The listing builds one solid part. Answer for the finished solid, in the listing's coordinates (mm). A direction names the side the tool comes from. Coordinates: 2 decimals unless noted, no trailing zeros. Loops run counter-clockwise (first coordinate to the right, second up) from the corner with the lowest first, then second, coordinate; pieces in that order, holes last. Notation, with made-up numbers: M 17,18 L 37,18 A14 ccw 37,25 Z; hole C -2,42 d1. An arc over 180 degrees is marked long. Answer as a JSON object with one key per item and string values. Group by question number.
1. A cutting plane is placed at B-B on y = 29.5. State how many separate pieces and enclosed holes the cut face has, and give its area (3 significant figures).
2. A cutting plane is placed at A-A on z = 18.5. Give the vertices of the cut face in (x, y), and give its area (3 significant figures).
3. Straight lines are drawn through the part: L1, parallel to X at y = 26.5, z = 9; L2, parallel to X at y = -19.5, z = 7.75 (1 decimal); L3, parallel to Y at x = -25, z = 1.75. For each, find the intervals that lie inside material, in ascending order.
4. For faces 1 (the face through (-14, 25, 2)), 2 (the face through (23.5, 0, 1)), determine the directions among +Z, -Z, +X, -X, +Y, -Y from which every point of the face is accessible in a straight line to the end or side of a thin tool.
5. Given pin 1 (1.5 mm diameter, centred on x = 16.5, z = 3.5, fed in from -Y); pin 2 (2.5 mm diameter, centred on x = 14, y = 23, fed in from -Z); pin 3 (5 mm diameter, centred on x = 21.5, y = -19.5, fed in from +Z); pin 4 (3 mm diameter, centred on x = 20.5, y = 2.5, fed in from -Z), each flat-ended and moving along its own axis, determine where each tip first touches the part or whether it passes through.
from build123d import *

# Parameters (mm, degrees)
SKETCH1_R                = 31.75
BOSS_EXTRUDE1_DEPTH      = 13
FILLET1_R                = 5
SHELL1_T                 = -1.5
SKETCH9_R                = 35.624492326
SKETCH9_R_2              = 27.25
BOSS_EXTRUDE5_DEPTH      = 2
SKETCH2_W                = 7.351458637
SKETCH2_H                = 15
BOSS_EXTRUDE2_DEPTH      = 2
BOSS_EXTRUDE3_REACH      = 59.839
SKETCH4_W                = 10.926622009
SKETCH4_H                = 2.5
FILLET3_R                = 1
BOSS_EXTRUDE4_REACH      = 60.696
BOSS_EXTRUDE4_END_RADIUS = 38.178049598
SKETCH5_W                = 10.787818312
SKETCH5_H                = 8
SKETCH6_W                = 2
SKETCH6_H                = 4
CUT_EXTRUDE1_DEPTH       = 4
SKETCH7_W                = 4
SKETCH7_H                = 2
CUT_EXTRUDE2_DEPTH       = 4
SKETCH8_W                = 4
SKETCH8_H                = 2
CUT_EXTRUDE3_DEPTH       = 4
FILLET5_R                = 1
CHAMFER2_SIZE            = 1.5
FILLET7_R                = 1
CHAMFER3_SIZE            = 0.5


with BuildPart() as part:
    # Sketch1 → Boss-Extrude1 (new body)
    with BuildSketch(Plane.XY):
        with Locations(Location((0, 0, 0), (0, 0, 180))):
            Circle(SKETCH1_R)
    extrude(amount=BOSS_EXTRUDE1_DEPTH)

    # Fillet1
    fillet1_edges = [part.edges().sort_by_distance(p)[0] for p in [
        (31.75, 0, 13),
    ]]
    fillet(fillet1_edges, radius=FILLET1_R)

    # Sketch12 → Revolve3 (revolve)
    with BuildSketch(Plane(origin=(0, 0, 0), x_dir=(1, 0, 0), z_dir=(0, 1, 0)), mode=Mode.PRIVATE) as revolve3_sk:
        with BuildLine():
            Line((0, -25.950011953), (0, -11.6))
            Line((0, -11.6), (27.242806288, -11.6))
            Line((27.242806288, -11.6), (27.242806288, -11.107193712))
            ThreePointArc((27.242806288, -11.107193712), (29.439924032, -10.197117744), (30.35, -8))
            Line((30.35, -8), (30.35, 0))
            Line((30.35, 0), (37.227524794, 0))
            ThreePointArc((37.227524794, 0), (22.689709797, -18.822303202), (0, -25.950011953))
        make_face()
    revolve(revolve3_sk.sketch.rotate(Axis((0, 0, 27.247512551), (0, 0, -1)), 180), axis=Axis((0, 0, 27.247512551), (0, 0, -1)))

    # Shell1
    shell1_openings = [part.faces().sort_by_distance(p)[0] for p in [
        (0, 0, 0),
    ]]
    offset(amount=SHELL1_T, openings=shell1_openings, kind=Kind.INTERSECTION)

    # Sketch9 → Boss-Extrude5 (add)
    with BuildSketch(Plane(origin=(0, 0, 0), x_dir=(-1, 0, 0), z_dir=(0, 0, -1))):
        Circle(SKETCH9_R)
        Circle(SKETCH9_R_2, mode=Mode.SUBTRACT)
    extrude(amount=-BOSS_EXTRUDE5_DEPTH)

    # Sketch2 → Boss-Extrude2 (add)
    with BuildSketch(Plane(origin=(0, 0, 0), x_dir=(-1, 0, 0), z_dir=(0, 0, -1))):
        with Locations((-27.175729319, 0)):
            Rectangle(SKETCH2_W, SKETCH2_H)
        Polygon((8.93053879, 30.468146923), (5.254809472, 24.101596989), (18.245190528, 16.601596989), (21.920919847, 22.968146923), align=None)
        Polygon((21.920919847, -22.968146923), (18.245190528, -16.601596989), (5.254809472, -24.101596989), (8.93053879, -30.468146923), align=None)
    extrude(amount=-BOSS_EXTRUDE2_DEPTH)

    # Sketch4 → Boss-Extrude3 (add, up to next)
    with BuildSketch(Plane.XY.offset(2), mode=Mode.PRIVATE) as boss_extrude3_sk1:
        with Locations((28.963311004, 6.25)):
            Rectangle(SKETCH4_W, SKETCH4_H)
    boss_extrude3_tool1 = extrude(boss_extrude3_sk1.sketch, amount=BOSS_EXTRUDE3_REACH, mode=Mode.PRIVATE) - part.part
    # Sketch4 → Boss-Extrude3 (add, up to next)
    with BuildSketch(Plane.XY.offset(2), mode=Mode.PRIVATE) as boss_extrude3_sk2:
        with Locations((28.963311004, -6.25)):
            Rectangle(SKETCH4_W, SKETCH4_H)
    boss_extrude3_tool2 = extrude(boss_extrude3_sk2.sketch, amount=BOSS_EXTRUDE3_REACH, mode=Mode.PRIVATE) - part.part
    # Sketch4 → Boss-Extrude3 (add, up to next)
    with BuildSketch(Plane.XY.offset(2), mode=Mode.PRIVATE) as boss_extrude3_sk3:
        Polygon((-16.080127019, -17.851596989), (-21.543438023, -27.314329226), (-23.708501533, -26.064329226), (-18.245190528, -16.601596989), align=None)
    boss_extrude3_tool3 = extrude(boss_extrude3_sk3.sketch, amount=BOSS_EXTRUDE3_REACH, mode=Mode.PRIVATE) - part.part
    # Sketch4 → Boss-Extrude3 (add, up to next)
    with BuildSketch(Plane.XY.offset(2), mode=Mode.PRIVATE) as boss_extrude3_sk4:
        Polygon((-7.419872981, -22.851596989), (-12.883183985, -32.314329226), (-10.718120476, -33.564329226), (-5.254809472, -24.101596989), align=None)
    boss_extrude3_tool4 = extrude(boss_extrude3_sk4.sketch, amount=BOSS_EXTRUDE3_REACH, mode=Mode.PRIVATE) - part.part
    # Sketch4 → Boss-Extrude3 (add, up to next)
    with BuildSketch(Plane.XY.offset(2), mode=Mode.PRIVATE) as boss_extrude3_sk5:
        Polygon((-7.419872981, 22.851596989), (-12.883183985, 32.314329226), (-10.718120476, 33.564329226), (-5.254809472, 24.101596989), align=None)
    boss_extrude3_tool5 = extrude(boss_extrude3_sk5.sketch, amount=BOSS_EXTRUDE3_REACH, mode=Mode.PRIVATE) - part.part
    # Sketch4 → Boss-Extrude3 (add, up to next)
    with BuildSketch(Plane.XY.offset(2), mode=Mode.PRIVATE) as boss_extrude3_sk6:
        Polygon((-16.080127019, 17.851596989), (-21.543438023, 27.314329226), (-23.708501533, 26.064329226), (-18.245190528, 16.601596989), align=None)
    boss_extrude3_tool6 = extrude(boss_extrude3_sk6.sketch, amount=BOSS_EXTRUDE3_REACH, mode=Mode.PRIVATE) - part.part
    add(boss_extrude3_tool1.solids().sort_by_distance((28.963311, 6.25, 2))[0])
    add(boss_extrude3_tool2.solids().sort_by_distance((28.963311, -6.25, 2))[0])
    add(boss_extrude3_tool3.solids().sort_by_distance((-19.894314, -21.957963, 2))[0])
    add(boss_extrude3_tool4.solids().sort_by_distance((-9.068997, -28.207963, 2))[0])
    add(boss_extrude3_tool5.solids().sort_by_distance((-9.068997, 28.207963, 2))[0])
    add(boss_extrude3_tool6.solids().sort_by_distance((-19.894314, 21.957963, 2))[0])

    # Fillet3
    fillet3_edges = [part.edges().sort_by_distance(p)[0] for p in [
        (23.5, -7.5, 7.705328032),
        (23.5, 7.5, 7.705328032),
        (-5.254809472, 24.101596989, 7.705328032),
        (-18.245190528, 16.601596989, 7.705328032),
        (-18.245190528, -16.601596989, 7.705328032),
        (-5.254809472, -24.101596989, 7.705328032),
    ]]
    fillet(fillet3_edges, radius=FILLET3_R)

    # Boss-Extrude4: up to this sphere (the profile starts inside it)
    boss_extrude4_end = Location((0, 0, -13.728037644)) * Sphere(BOSS_EXTRUDE4_END_RADIUS, mode=Mode.PRIVATE)
    # Sketch5 → Boss-Extrude4 (add, up to the surface)
    with BuildSketch(Plane(origin=(0, 0, 0), x_dir=(-1, 0, 0), z_dir=(0, 0, -1)), mode=Mode.PRIVATE) as boss_extrude4_sk1:
        with Locations((29.393909156, 0)):
            Rectangle(SKETCH5_W, SKETCH5_H)
    boss_extrude4_tool1 = extrude(boss_extrude4_sk1.sketch, amount=-BOSS_EXTRUDE4_REACH, mode=Mode.PRIVATE) & boss_extrude4_end
    add(boss_extrude4_tool1.solids().sort_by_distance((-29.393909, 0, 0))[0])
    # Sketch5 → Boss-Extrude4 (add, up to the surface)
    with BuildSketch(Plane(origin=(0, 0, 0), x_dir=(-1, 0, 0), z_dir=(0, 0, -1)), mode=Mode.PRIVATE) as boss_extrude4_sk2:
        Polygon((-8.535898385, -22.784609691), (-15.464101615, -18.784609691), (-20.858010771, -28.127134401), (-13.929807541, -32.127134401), align=None)
    boss_extrude4_tool2 = extrude(boss_extrude4_sk2.sketch, amount=-BOSS_EXTRUDE4_REACH, mode=Mode.PRIVATE) & boss_extrude4_end
    add(boss_extrude4_tool2.solids().sort_by_distance((14.696955, -25.455872, 0))[0])
    # Sketch5 → Boss-Extrude4 (add, up to the surface)
    with BuildSketch(Plane(origin=(0, 0, 0), x_dir=(-1, 0, 0), z_dir=(0, 0, -1)), mode=Mode.PRIVATE) as boss_extrude4_sk3:
        Polygon((-15.464101615, 18.784609691), (-8.535898385, 22.784609691), (-13.929807541, 32.127134401), (-20.858010771, 28.127134401), align=None)
    boss_extrude4_tool3 = extrude(boss_extrude4_sk3.sketch, amount=-BOSS_EXTRUDE4_REACH, mode=Mode.PRIVATE) & boss_extrude4_end
    add(boss_extrude4_tool3.solids().sort_by_distance((14.696955, 25.455872, 0))[0])

    # Sketch6 → Cut-Extrude1 (cut)
    with BuildSketch(Plane(origin=(-24, 0, 0), x_dir=(0, 0, -1), z_dir=(1, 0, 0))):
        with Locations((-6, 0)):
            Rectangle(SKETCH6_W, SKETCH6_H)
    extrude(amount=-CUT_EXTRUDE1_DEPTH, mode=Mode.SUBTRACT)

    # Sketch7 → Cut-Extrude2 (cut)
    with BuildSketch(Plane(origin=(12, -20.784609691, 0), x_dir=(0.8660254037844365, 0.5000000000000039, 0), z_dir=(-0.5000000000000038, 0.8660254037844364, 0))):
        with Locations((0, -6)):
            Rectangle(SKETCH7_W, SKETCH7_H)
    extrude(amount=-CUT_EXTRUDE2_DEPTH, mode=Mode.SUBTRACT)

    # Sketch8 → Cut-Extrude3 (cut)
    with BuildSketch(Plane(origin=(12, 20.784609691, 0), x_dir=(0.8660254037844257, -0.5000000000000224, 0), z_dir=(-0.5000000000000224, -0.8660254037844258, 0))):
        with Locations((0, 6)):
            Rectangle(SKETCH8_W, SKETCH8_H)
    extrude(amount=-CUT_EXTRUDE3_DEPTH, mode=Mode.SUBTRACT)

    # Fillet5
    fillet5_edges = [part.edges().sort_by_distance(p)[0] for p in [
        (-24, -4, 7.846211216),
        (-24, 4, 7.846211216),
        (15.464101615, -18.784609691, 7.846211216),
        (8.535898385, -22.784609691, 7.846211216),
        (8.535898385, 22.784609691, 7.846211216),
        (15.464101615, 18.784609691, 7.846211216),
    ]]
    fillet(fillet5_edges, radius=FILLET5_R)

    # Chamfer2
    # the kernel refuses this chamfer: 1.5, 1.168019183 mm, written as the material it takes off along each edge
    with BuildSketch(Plane(origin=(0, 0, 0), x_dir=(-1, 0, 0), z_dir=(0, -1, 0))) as chamfer2_piece_1:
        with BuildLine():
            Line((37.227524794 - CHAMFER2_SIZE, 0), (36.810195939, -1.082671144))
            ThreePointArc((36.810195939, -1.082671144), (37.018444042, -0.554203797), (37.227524794, 0))
            Line((37.227524794, 0), (37.227524794 - CHAMFER2_SIZE, 0))
        make_face()
    revolve(axis=Axis((0, 0, 0), (0, 0, -1)), mode=Mode.SUBTRACT)

    # Fillet7
    fillet7_edges = [part.edges().sort_by_distance(p)[0] for p in [
        (36.810195939, 0, 1.082671144),
    ]]
    fillet(fillet7_edges, radius=FILLET7_R)

    # Chamfer3
    chamfer3_edges = [part.edges().sort_by_distance(p)[0] for p in [
        (-11.75, 20.351596989, 0),
        (-11.75, -20.351596989, 0),
        (-6.179201142, -25.702690328, 0),
        (23.5, 0, 0),
        (25.34878334, 7.5, 0),
        (-19.169582199, 18.202690328, 0),
        (-5.654909049, -24.208803348, 0),
        (-18.13798417, -17.001696566, 0),
        (23.792893219, -7.207106781, 0),
        (23.792893219, 7.207106781, 0),
        (-5.654909049, 24.208803348, 0),
        (-18.13798417, 17.001696566, 0),
        (25.34878334, -7.5, 0),
        (-6.179201142, 25.702690328, 0),
        (-19.169582199, -18.202690328, 0),
    ]]
    chamfer(chamfer3_edges, length=CHAMFER3_SIZE)


solid = part.part
From the geometry:
{
 "1": {"separate pieces": "1", "enclosed holes": "2", "area": "226 mm²"},
 "2": {"outline": "C 0,0 d46.29; hole C 0,0 d40.93", "area": "367 mm²"},
 "3": {"L1": "x = -18.86 to -15.45, -9.53 to -6.64, 10.68 to 18.86", "L2": "x = -27.1 to -24.8, -19.9 to -17, 14.2 to 15.9, 24.8 to 27.1", "L3": "y = -26.64 to -10.84, -4 to 4, 10.84 to 26.64"},
 "4": {"face 1": "none", "face 2": "-Z"},
 "5": {"pin 1": "stops at y = -32.26", "pin 2": "stops at z = 0", "pin 3": "stops at z = 15.78", "pin 4": "stops at z = 17.37"}
}
